The drawing under review shows one solid part. Ordinate dimensions are in mm from its lowest x, y, z. Give positions to 0.01 mm unless a question says otherwise; leave off trailing zeros. Write each loop counter-clockwise with the first axis right and the second up, starting at its lowest first coordinate (ties: lowest second). Pieces come first, ordered by that corner, then holes.
Q1. Mouldability with a two-part tool opening along Z and no side actions: class the marked faces 1, 2 and 3 as released by +Z, released by -Z, zero draft, split by the parting line, or undercut.
Q2. We need section A-A (x = 1.9). Write out the cut boundary in (y, z) (1 decimal).
Q3. Insertion check: P1, Ø2, axis at y = 18, z = 12, coming from the +X side; P2, Ø1, axis at x = 3, z = 3.5, coming from the -Y side (1 decimal). Each pin has a flat end and moves straight along its axis. Give the tip position at first contact, or say it passes through.
Q4. For line 1 (Z direction, x = 0.95, y = 7.5); line 2 (Z direction, x = 1.85, y = 11); line 3 (Y direction, x = 1.45, z = 4) (1 decimal), list the stretches that pass through material, from the lowest coordinate up.
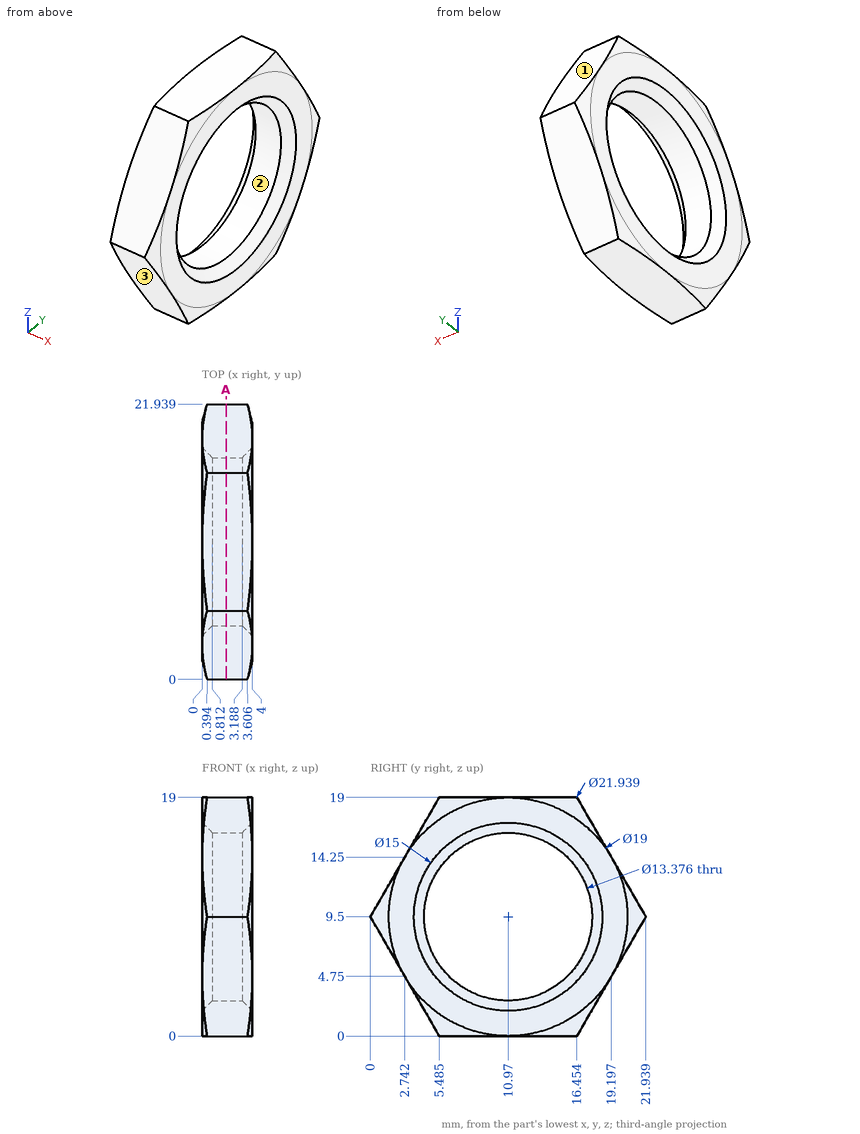
Computed:
1. face 1: released by +Z
1. face 2: undercut
1. face 3: released by -Z
2. outline: (0, 9.5) - (5.5, 0) - (16.5, 0) - (21.9, 9.5) - (16.5, 19) - (5.5, 19) - close; hole circle Ø13.4 at (11, 9.5)
3. P1: stops at x = 4
3. P2: stops at y = 3.2
4. line 1: z = 0 to 3.78, 15.22 to 19
4. line 2: z = 0 to 2.81, 16.19 to 19
4. line 3: y = 3.2 to 7.2, 14.8 to 18.8
